The model under review builds one solid part; all positions refer to its coordinate system, in mm. A direction names the side the tool comes from. Round coordinates to 2 decimals unless told otherwise and drop trailing zeros. Loops run counter-clockwise (first coordinate to the right, second up) from the corner with the lowest first, then second, coordinate; pieces in that order, holes last. Notation, with made-up numbers: M -22,64.25 L 30,64.25 A28 ccw 30,100.25 Z; hole C 5.25,18 d4. An arc over 180 degrees is marked long. Answer as a JSON object with one key per item and string values. Group by question number.
Item 1: Consider section A-A (y = 8). Give the boundary of the cut face in (x, z), and give its area (3 significant figures).
Item 2: To check wall thickness, follow line 1 (Y direction, x = 4, z = -5.25); line 2 (Y direction, x = 0.25, z = 0.5); line 3 (Z direction, x = 3.25, y = 4.75). State the ranges of each line that lie inside material, in increasing order.
Item 3: Insertion check: P1, Ø2, axis at x = 1.5, z = -1.5, coming from the +Y side; P2, Ø5, axis at y = 16.5, z = 2.5, coming from the -X side. Each pin has a flat end and moves straight along its axis. Give the tip position at first contact, or say it passes through.
Item 4: Tool access review of faces 1 (the face through (0, 0, 0)), 2 (the face through (-1, 18, 0)): name each direction out of +Z, -Z, +X, -X, +Y, -Y from which nothing blocks a thin tool from reaching the whole face with its end or side.
Item 5: Consider section B-B (y = 25). Give the boundary of the cut face in (x, z).
```python
from build123d import *

# Parameters (mm, degrees)
SKETCH1_R           = 9
BOSS_EXTRUDE1_DEPTH = 5
SKETCH2_R           = 7.15
BOSS_EXTRUDE2_DEPTH = 5
SKETCH3_R           = 1
BOSS_EXTRUDE3_DEPTH = 16.8
FILLET1_R           = 2.5
CHAMFER1_SIZE       = 1


with BuildPart() as part:
    # Sketch1 → Boss-Extrude1 (new body)
    with BuildSketch(Plane(origin=(0, 0, 0), x_dir=(1, 0, 0), z_dir=(0, 1, 0))):
        with Locations(Location((0, 0, 0), (0, 0, 270))):
            Circle(SKETCH1_R)
    extrude(amount=BOSS_EXTRUDE1_DEPTH)

    # Sketch2 → Boss-Extrude2 (add)
    with BuildSketch(Plane(origin=(0, 5, 0), x_dir=(1, 0, 0), z_dir=(0, 1, 0))):
        with Locations(Location((0, 0, 0), (0, 0, 270))):
            Circle(SKETCH2_R)
    extrude(amount=BOSS_EXTRUDE2_DEPTH)

    # Sketch3 → Boss-Extrude3 (add)
    with BuildSketch(Plane(origin=(0, 10, 0), x_dir=(1, 0, 0), z_dir=(0, 1, 0))):
        with Locations(Location((0, 0, 0), (0, 0, 270))):
            Circle(SKETCH3_R)
    extrude(amount=BOSS_EXTRUDE3_DEPTH)

    # Fillet1
    # the kernel refuses this fillet: 2.5 mm, written as the material it takes off along each edge
    with BuildSketch(Plane(origin=(0, 0, 0), x_dir=(0, 0, 1), z_dir=(-1, 0, 0))) as fillet1_piece_1:
        with BuildLine():
            CenterArc((9 - FILLET1_R, FILLET1_R), FILLET1_R, 270, 90)
            Line((9 - FILLET1_R, 0), (9 - FILLET1_R, -FILLET1_R * 0.02))
            Line((9 - FILLET1_R, -FILLET1_R * 0.02), (9 + FILLET1_R * 0.02, -FILLET1_R * 0.02))
            Line((9 + FILLET1_R * 0.02, -FILLET1_R * 0.02), (9 + FILLET1_R * 0.02, FILLET1_R))
            Line((9 + FILLET1_R * 0.02, FILLET1_R), (9, FILLET1_R))
        make_face()
    revolve(axis=Axis((0, 0, 0), (0, 1, 0)), mode=Mode.SUBTRACT)
    with BuildSketch(Plane(origin=(0, 5, 0), x_dir=(0, 0, 1), z_dir=(-1, 0, 0))) as fillet1_piece_2:
        with BuildLine():
            CenterArc((6.5, -2.414021541), FILLET1_R, 0, 74.929937855)
            Line((7.15, 0), (7.163, 0.048280431))
            ThreePointArc((7.163, 0.048280431), (8.075, 0.05), (9, 0.05))
            Line((9, 0.05), (9.05, 0))
            Line((9.05, 0), (9.05, -2.414021541))
            Line((9.05, -2.414021541), (9, -2.414021541))
        make_face()
    revolve(axis=Axis((0, 5, 0), (0, 1, 0)), mode=Mode.SUBTRACT)

    # Chamfer1
    chamfer1_edges = [part.edges().sort_by_distance(p)[0] for p in [
        (0, 26.8, -1),
    ]]
    chamfer(chamfer1_edges, length=CHAMFER1_SIZE)


solid = part.part
```
Geometry results:
{
 "1": {"outline": "C 0,0 d14.3", "area": "161 mm^2"},
 "2": {"line 1": "y = 0 to 10", "line 2": "y = 0 to 26.24", "line 3": "z = -7.04 to 7.04"},
 "3": {"P1": "stops at y = 10", "P2": "stops at x = -1"},
 "4": {"face 1": "+Z, -Z, +X, -X, -Y", "face 2": "+Y"},
 "5": {"outline": "C 0,0 d2"}
}
